Source: CAD feature listing. Evaluate the final solid. Frame: model axes, mm. A direction names the side the tool comes from. Give positions to 0.01 mm unless a question says otherwise; leave off trailing zeros. Order: outer loops, then holes, each group sorted by start corner. A loop starts at its lowest first (then second) coordinate and runs counter-clockwise, first axis right, second up. Notation, with made-up numbers: (12, 24.5) -> (24, 24.5) arc R17 cw to (24, 46.5) -> close; hole circle Ø8 at (89.25, 28). An arc over 180 degrees is marked (long way). Use one line per item in the form item = value. Start each with the question number.
from build123d import *

# Parameters (mm, degrees)
SKETCH1_R                = 30
SKETCH1_W                = 35
SKETCH1_H                = 5
SKETCH1_H_2              = 28
BOSS_EXTRUDE1_DEPTH      = 10
SKETCH2_W                = 35
SKETCH2_H                = 44.33
SKETCH2_R                = 5.5
BOSS_EXTRUDE2_DEPTH      = 19
BOSS_EXTRUDE2_DEPTH_BACK = 19
SKETCH2_4_R              = 4
SKETCH2_4_W              = 35
SKETCH2_4_H              = 44.33
SKETCH2_4_R_2            = 5.5
CUT_EXTRUDE1_DEPTH       = 14
SKETCH3_W                = 35
SKETCH3_H                = 30
SKETCH3_R                = 5.5
BOSS_EXTRUDE3_DEPTH      = 19
SKETCH3_3_R              = 4
SKETCH3_3_W              = 35
SKETCH3_3_H              = 30
SKETCH3_3_R_2            = 5.5
CUT_EXTRUDE2_DEPTH       = 14
SKETCH2_5_R              = 5.5
SKETCH2_5_R_2            = 4
BOSS_EXTRUDE4_DEPTH      = 19
SKETCH2_6_R              = 5.5
SKETCH2_6_R_2            = 4
CUT_EXTRUDE3_DEPTH       = 6
SKETCH3_4_R              = 5.5
SKETCH3_4_R_2            = 4
BOSS_EXTRUDE5_DEPTH      = 19
SKETCH3_5_R              = 5.5
SKETCH3_5_R_2            = 4
CUT_EXTRUDE4_DEPTH       = 6
SKETCH5_R                = 4
BOSS_EXTRUDE6_DEPTH      = 19
CUT_EXTRUDE5_DEPTH       = 14
SKETCH5_6_R              = 5.5
SKETCH5_6_R_2            = 4
CUT_EXTRUDE6_DEPTH       = 6


with BuildPart() as part:
    # Sketch1 → Boss-Extrude1 (new body)
    with BuildSketch(Plane(origin=(0, 580, 0), x_dir=(1, 0, 0), z_dir=(0, 1, 0))):
        Polygon((677.75, 14), (692.03, 14), (692.03, 9), (692.03, -19), (692.03, -24), (727.03, -24), (727.03, -19), (727.03, 9), (727.03, 14), (757.75, 14), (757.75, -224), (755.84, -224), (755.84, -219), (755.84, -191), (755.84, -186), (720.84, -186), (720.84, -191), (720.84, -219), (720.84, -224), (677.75, -224), align=None)
        with Locations((717.75, -110)):
            Circle(SKETCH1_R, mode=Mode.SUBTRACT)
        with Locations((709.53, 11.5)):
            Rectangle(SKETCH1_W, SKETCH1_H)
        with Locations((709.53, -5)):
            Rectangle(SKETCH1_W, SKETCH1_H_2)
        with Locations((709.53, -21.5)):
            Rectangle(SKETCH1_W, SKETCH1_H)
        with Locations((738.34, -188.5)):
            Rectangle(SKETCH1_W, SKETCH1_H)
        with Locations((738.34, -205)):
            Rectangle(SKETCH1_W, SKETCH1_H_2)
        with Locations((738.34, -221.5)):
            Rectangle(SKETCH1_W, SKETCH1_H)
    extrude(amount=BOSS_EXTRUDE1_DEPTH)

    # Sketch2 → Boss-Extrude2 (add, two sides)
    with BuildSketch(Plane.XY.offset(205)) as boss_extrude2_sk:
        with Locations((738.34, 557.835)):
            Rectangle(SKETCH2_W, SKETCH2_H)
        with Locations((738.34, 550.67)):
            Circle(SKETCH2_R, mode=Mode.SUBTRACT)
    extrude(amount=BOSS_EXTRUDE2_DEPTH)
    extrude(boss_extrude2_sk.sketch, amount=-BOSS_EXTRUDE2_DEPTH_BACK)

    # Sketch2<4> → Cut-Extrude1 (cut, symmetric)
    with BuildSketch(Plane.XY.offset(205)):
        with Locations((738.34, 550.67)):
            Circle(SKETCH2_4_R)
        with Locations((738.34, 557.835)):
            Rectangle(SKETCH2_4_W, SKETCH2_4_H)
        with Locations((738.34, 550.67)):
            Circle(SKETCH2_4_R_2, mode=Mode.SUBTRACT)
    extrude(amount=CUT_EXTRUDE1_DEPTH, both=True, mode=Mode.SUBTRACT)

    # Sketch3 → Boss-Extrude3 (add, symmetric)
    with BuildSketch(Plane.XY.offset(5)):
        with Locations((709.53, 565)):
            Rectangle(SKETCH3_W, SKETCH3_H)
        with Locations((709.53, 565)):
            Circle(SKETCH3_R, mode=Mode.SUBTRACT)
    extrude(amount=BOSS_EXTRUDE3_DEPTH, both=True)

    # Sketch3<3> → Cut-Extrude2 (cut, symmetric)
    with BuildSketch(Plane.XY.offset(5)):
        with Locations((709.53, 565)):
            Circle(SKETCH3_3_R)
        with Locations((709.53, 565)):
            Rectangle(SKETCH3_3_W, SKETCH3_3_H)
        with Locations((709.53, 565)):
            Circle(SKETCH3_3_R_2, mode=Mode.SUBTRACT)
    extrude(amount=CUT_EXTRUDE2_DEPTH, both=True, mode=Mode.SUBTRACT)

    # Sketch2<5> → Boss-Extrude4 (add, symmetric)
    with BuildSketch(Plane.XY.offset(205)):
        with Locations((738.34, 550.67)):
            Circle(SKETCH2_5_R)
        with Locations((738.34, 550.67)):
            Circle(SKETCH2_5_R_2, mode=Mode.SUBTRACT)
    extrude(amount=BOSS_EXTRUDE4_DEPTH, both=True)

    # Sketch2<6> → Cut-Extrude3 (cut, symmetric)
    with BuildSketch(Plane.XY.offset(205)):
        with Locations((738.34, 550.67)):
            Circle(SKETCH2_6_R)
        with Locations((738.34, 550.67)):
            Circle(SKETCH2_6_R_2, mode=Mode.SUBTRACT)
    extrude(amount=CUT_EXTRUDE3_DEPTH, both=True, mode=Mode.SUBTRACT)

    # Sketch3<4> → Boss-Extrude5 (add, symmetric)
    with BuildSketch(Plane.XY.offset(5)):
        with Locations((709.53, 565)):
            Circle(SKETCH3_4_R)
        with Locations((709.53, 565)):
            Circle(SKETCH3_4_R_2, mode=Mode.SUBTRACT)
    extrude(amount=BOSS_EXTRUDE5_DEPTH, both=True)

    # Sketch3<5> → Cut-Extrude4 (cut, symmetric)
    with BuildSketch(Plane.XY.offset(5)):
        with Locations((709.53, 565)):
            Circle(SKETCH3_5_R)
        with Locations((709.53, 565)):
            Circle(SKETCH3_5_R_2, mode=Mode.SUBTRACT)
    extrude(amount=CUT_EXTRUDE4_DEPTH, both=True, mode=Mode.SUBTRACT)

    # Sketch5 → Boss-Extrude6 (add, symmetric)
    with BuildSketch(Plane.XY.offset(49.7)):
        with BuildLine():
            Line((677.75, 580), (677.75, 590))
            Line((677.75, 590), (612.765312184, 529.288994825))
            ThreePointArc((612.765312184, 529.288994825), (612.586521385, 521.425816604), (620.451731788, 521.424030013))
            Line((620.451731788, 521.424030013), (677.75, 580))
        make_face()
        with Locations((616.52, 525.27)):
            Circle(SKETCH5_R, mode=Mode.SUBTRACT)
    extrude(amount=BOSS_EXTRUDE6_DEPTH, both=True)

    # Sketch5<5> → Cut-Extrude5 (cut, symmetric)
    with BuildSketch(Plane.XY.offset(49.7)):
        with BuildLine():
            Line((677.75, 580), (677.75, 590))
            Line((677.75, 590), (612.765312184, 529.288994825))
            ThreePointArc((612.765312184, 529.288994825), (618.710800882, 530.314838104), (622.02, 525.27))
            ThreePointArc((622.02, 525.27), (621.612863872, 523.193286832), (620.451731788, 521.424030013))
            Line((620.451731788, 521.424030013), (677.75, 580))
        make_face()
    extrude(amount=CUT_EXTRUDE5_DEPTH, both=True, mode=Mode.SUBTRACT)

    # Sketch5<6> → Cut-Extrude6 (cut, symmetric)
    with BuildSketch(Plane.XY.offset(49.7)):
        with Locations((616.52, 525.27)):
            Circle(SKETCH5_6_R)
        with Locations((616.52, 525.27)):
            Circle(SKETCH5_6_R_2, mode=Mode.SUBTRACT)
    extrude(amount=CUT_EXTRUDE6_DEPTH, both=True, mode=Mode.SUBTRACT)


solid = part.part
1) Reachability of faces 5 (the face through (677.75, 585, 9)), 6 (the face through (720.84, 558, 222)), 7 (the face through (727.03, 565, 22)), 8 (the face through (709, 550, 22)) from +Z, -Z, +X, -X, +Y, -Y: full face, straight path, thin tool, end or side. Return the list, or none.
2) Cut plane A-A, the plane z = 105. Return the cut outline in (x, y), plus the area to 3 significant figures.
3) Cut plane D-D, the plane y = 584. Return the cut outline in (x, z), plus the area to 3 significant figures.
4) Cut plane B-B, the plane x = 616.52. Return the cut outline in (y, z), plus the area to 3 significant figures.
5) Pin query (flat end, axial travel): pin 1 (1 mm diameter, centred on x = 641, y = 542, fed in from +Z); pin 2 (5.5 mm diameter, centred on y = 565.5, z = -12, fed in from -X); pin 3 (8 mm diameter, centred on x = 705, y = 543, fed in from -Z); pin 4 (5.5 mm diameter, centred on y = 562.5, z = 222.5, fed in from +X). Return the tip coordinate at first contact, or that it passes through.
6) Material intervals for probe 1 along Y at (x, z) = (709, 16); probe 2 along X at (y, z) = (525, 61); probe 3 along X at (y, z) = (565, 21), sorted ascending.
7) Draft query along Z for faces 1 (the face through (755.84, 558, 189)), 2 (the face through (644, 552, 68.7)), 3 (the face through (648, 556, 63.7)), 4 (the face through (734.3, 554.4, 215.1)). Return one class per face: +Z half, -Z half, draft (parallel to the pull), parting line (faces both ways), or undercut.
8) Cut plane C-C, the plane x = 638. Return the cut outline in (y, z).
Output values:
q1.face_5 = -Z, -X, +Y, -Y
q1.face_6 = +Z, -X, -Y
q1.face_7 = -Z, +X, -Y
q1.face_8 = -Z, +X, -X, -Y
q2.outline = (677.75, 580) -> (688.17, 580) -> (688.17, 590) -> (677.75, 590) -> close; (747.33, 580) -> (757.75, 580) -> (757.75, 590) -> (747.33, 590) -> close
q2.area = 208 mm^2
q3.outline = (671.33, 30.7) -> (677.75, 30.7) -> (677.75, -14) -> (757.75, -14) -> (757.75, 224) -> (677.75, 224) -> (677.75, 68.7) -> (671.33, 68.7) -> (671.33, 63.7) -> (677.75, 63.7) -> (677.75, 35.7) -> (671.33, 35.7) -> close; hole circle Ø60 at (717.75, 110)
q3.area = 16,300 mm^2
q4.outline = (519.77, 30.7) -> (521.27, 30.7) -> (521.27, 43.7) -> (519.77, 43.7) -> close; (519.77, 55.7) -> (521.27, 55.7) -> (521.27, 68.7) -> (519.77, 68.7) -> close; (529.27, 30.7) -> (532.8, 30.7) -> (532.8, 35.7) -> (530.77, 35.7) -> (530.77, 43.7) -> (529.27, 43.7) -> close; (529.27, 55.7) -> (530.77, 55.7) -> (530.77, 63.7) -> (532.8, 63.7) -> (532.8, 68.7) -> (529.27, 68.7) -> close
q4.area = 98.3 mm^2
q5.pin_1 = 68.7
q5.pin_2 = 692.03
q5.pin_3 = through
q5.pin_4 = 755.84
q6.probe_1 = 559.53 to 561.04, 568.96 to 570.47, 580 to 590
q6.probe_2 = 611.03 to 612.53, 620.51 to 622.01
q6.probe_3 = 692.03 to 705.53, 713.53 to 727.03
q7.face_1 = draft
q7.face_2 = +Z half
q7.face_3 = undercut
q7.face_4 = undercut
q8.outline = (539.36, 30.7) -> (552.86, 30.7) -> (552.86, 35.7) -> (539.36, 35.7) -> close; (539.36, 63.7) -> (552.86, 63.7) -> (552.86, 68.7) -> (539.36, 68.7) -> close
